from build123d import *

# Parameters (mm, degrees)
SKETCH1_R           = 3.175
BOSS_EXTRUDE1_DEPTH = 3.175
SKETCH2_R           = 14.2875
CUT_EXTRUDE1_DEPTH  = 4.175
SKETCH4_R           = 6.35
SKETCH4_R_2         = 3.175
CUT_EXTRUDE2_DEPTH  = 4.175
SKETCH8_W           = 38.1
SKETCH8_H           = 100.0125
CUT_EXTRUDE3_DEPTH  = 4.175
SKETCH10_W          = 60.325
SKETCH10_H          = 48.559243464
CUT_EXTRUDE5_DEPTH  = 4.175
FILLET2_R           = 9.525


with BuildPart() as part:
    # Sketch1 → Boss-Extrude1 (new body)
    with BuildSketch(Plane.XY):
        with BuildLine():
            Line((-35.603982701, 119.957272705), (-127, -119.957272705))
            Line((-127, -119.957272705), (127, -119.957272705))
            Line((127, -119.957272705), (35.603982701, 119.957272705))
            ThreePointArc((35.603982701, 119.957272705), (0, 144.493850724), (-35.603982701, 119.957272705))
        make_face()
        with Locations((-25.4, 106.393850724)):
            Circle(SKETCH1_R, mode=Mode.SUBTRACT)
        with Locations((25.4, 106.393850724)):
            Circle(SKETCH1_R, mode=Mode.SUBTRACT)
    extrude(amount=BOSS_EXTRUDE1_DEPTH)

    # Sketch2 → Cut-Extrude1 (cut, through all)
    with BuildSketch(Plane.XY.offset(3.175)):
        with Locations((0, 106.393850724)):
            Circle(SKETCH2_R)
    extrude(amount=-CUT_EXTRUDE1_DEPTH, mode=Mode.SUBTRACT)

    # Sketch4 → Cut-Extrude2 (cut, through all)
    with BuildSketch(Plane.XY.offset(3.175)):
        with Locations((108.571571229, -107.257272705)):
            Circle(SKETCH4_R)
        with Locations((-76.2, -107.257272705)):
            Circle(SKETCH4_R_2)
        with Locations((19.05, -107.257272705)):
            Circle(SKETCH4_R_2)
    extrude(amount=-CUT_EXTRUDE2_DEPTH, mode=Mode.SUBTRACT)

    # Sketch8 → Cut-Extrude3 (cut, through all)
    with BuildSketch(Plane(origin=(0, 0, 0), x_dir=(-1, 0, 0), z_dir=(0, 0, -1))):
        with Locations((107.95, -69.951022705)):
            Rectangle(SKETCH8_W, SKETCH8_H)
    extrude(amount=-CUT_EXTRUDE3_DEPTH, mode=Mode.SUBTRACT)

    # Sketch10 → Cut-Extrude5 (cut, through all)
    with BuildSketch(Plane.XY.offset(3.175)):
        with BuildLine():
            Line((-9.525, 69.503684351), (-9.525, -14.248029241))
            Line((-9.525, -14.248029241), (-66.344311715, -14.248029241))
            Line((-66.344311715, -14.248029241), (-29.548259348, 82.34160822))
            ThreePointArc((-29.548259348, 82.34160822), (-20.56411854, 74.320075944), (-9.525, 69.503684351))
        make_face()
        with Locations((-39.6875, -57.577650973)):
            Rectangle(SKETCH10_W, SKETCH10_H)
        Polygon((9.525, -33.298029241), (9.525, -81.857272705), (92.100213987, -81.857272705), (73.601454572, -33.298029241), align=None)
        with BuildLine():
            Line((9.525, -14.248029241), (66.344311715, -14.248029241))
            Line((66.344311715, -14.248029241), (29.548259348, 82.34160822))
            ThreePointArc((29.548259348, 82.34160822), (20.56411854, 74.320075944), (9.525, 69.503684351))
            Line((9.525, 69.503684351), (9.525, -14.248029241))
        make_face()
    extrude(amount=-CUT_EXTRUDE5_DEPTH, mode=Mode.SUBTRACT)

    # Fillet2
    fillet2_edges = [part.edges().sort_by_distance(p)[0] for p in [
        (-29.548259348, 82.34160822, 1.5875),
        (-9.525, 69.503684351, 1.5875),
        (-9.525, -14.248029241, 1.5875),
        (-66.344311715, -14.248029241, 1.5875),
        (-69.85, -33.298029241, 1.5875),
        (-9.525, -33.298029241, 1.5875),
        (-9.525, -81.857272705, 1.5875),
        (-69.85, -81.857272705, 1.5875),
        (9.525, -33.298029241, 1.5875),
        (73.601454572, -33.298029241, 1.5875),
        (92.100213987, -81.857272705, 1.5875),
        (9.525, -81.857272705, 1.5875),
        (9.525, -14.248029241, 1.5875),
        (9.525, 69.503684351, 1.5875),
        (29.548259348, 82.34160822, 1.5875),
        (66.344311715, -14.248029241, 1.5875),
    ]]
    fillet(fillet2_edges, radius=FILLET2_R)


solid = part.part
Verification items for the finished model (mm, model axes). A direction names the side the tool comes from. Coordinates: 2 decimals unless noted, no trailing zeros. Loops run counter-clockwise (first coordinate to the right, second up) from the corner with the lowest first, then second, coordinate; pieces in that order, holes last. Notation, with made-up numbers: (83.25, 39) -> (102.25, 39) arc R24 cw to (102.25, 67) -> close; hole circle Ø1 at (-18.5, 31). An arc over 180 degrees is marked (long way). Answer as a JSON object with one key per item and string values. Group by question number.
Item 1: Tool access check on faces 1 (the flat face through (-6, -15, 0)), 2 (the cylindrical face through (-28.403, 75.255, 1.565)). Record the directions out of +Z, -Z, +X, -X, +Y, -Y that give a thin tool (end or side, any length) a straight path to the whole face; none if there is none.
Item 2: Sectioned sample at D-D on y = 6.5. Record the boundary of the cut face in (x, z) (3 decimals), plus the area to 3 significant figures.
Item 3: Depth check by flat-ended pin: pin 1 (1.6 mm diameter, centred on y = -56.5, z = 2, fed in from +X); pin 2 (1 mm diameter, centred on y = 43.5, z = 1.5, fed in from -X); pin 3 (1.5 mm diameter, centred on y = -19.5, z = 1, fed in from +X). Enter the tip coordinate at first touch or a pass-through.
Item 4: Sectioned sample at B-B on x = 25.5. Record the boundary of the cut face in (y, z) (3 decimals).
Item 5: Mould release check, pull along X, two halves, no side actions. Record for faces 3 (the cylindrical face through (0.64, 144.49, 1.57)), 4 (the flat face through (81.94, -1.68, 1.57)), 5 (the flat face through (48.11, 33.62, 1.61)): +X half, -X half, draft (parallel to the pull), parting line (faces both ways), or undercut.
Item 6: Scan lines: probe 1 along Y at (x, z) = (25.4, 1.3); probe 2 along X at (y, z) = (-11, 1.3); probe 3 along X at (y, z) = (-79, 0.8). Record each from-to range of solid material in increasing order.
Item 7: Sectioned sample at C-C on x = -76.2. Record the boundary of the cut face in (y, z) (3 decimals).
Item 8: Sectioned sample at A-A on y = -50. Record the boundary of the cut face in (x, z) (3 decimals).
Evaluation:
{
 "1": {"face 1": "-Z, +X, -X, +Y, -Y", "face 2": "+Z, -Z"},
 "2": {"outline": "(-78.826, 0) -> (-58.44, 0) -> (-58.44, 3.175) -> (-78.826, 3.175) -> close; (-9.525, 0) -> (9.525, 0) -> (9.525, 3.175) -> (-9.525, 3.175) -> close; (58.44, 0) -> (78.826, 0) -> (78.826, 3.175) -> (58.44, 3.175) -> close", "area": "190 mm²"},
 "3": {"pin 1": "stops at x = 103.13", "pin 2": "stops at x = -64.92", "pin 3": "stops at x = 89.02"},
 "4": {"outline": "(-119.957, 0) -> (-81.857, 0) -> (-81.857, 3.175) -> (-119.957, 3.175) -> close; (-33.298, 0) -> (-14.248, 0) -> (-14.248, 3.175) -> (-33.298, 3.175) -> close; (75.704, 0) -> (103.22, 0) -> (103.22, 3.175) -> (75.704, 3.175) -> close; (109.567, 0) -> (134.702, 0) -> (134.702, 3.175) -> (109.567, 3.175) -> close"},
 "5": {"face 3": "parting line", "face 4": "+X half", "face 5": "undercut"},
 "6": {"probe 1": "y = -119.96 to -81.86, -33.3 to -14.25, 75.7 to 103.22, 109.57 to 134.79", "probe 2": "x = -85.49 to -59.69, -11.89 to 11.89, 59.69 to 85.49", "probe 3": "x = -88.9 to -67.13, -12.25 to 12.25, 85.08 to 111.4"},
 "7": {"outline": "(-119.957, 0) -> (-110.432, 0) -> (-110.432, 3.175) -> (-119.957, 3.175) -> close; (-104.082, 0) -> (13.393, 0) -> (13.393, 3.175) -> (-104.082, 3.175) -> close"},
 "8": {"outline": "(-88.9, 0) -> (-69.85, 0) -> (-69.85, 3.175) -> (-88.9, 3.175) -> close; (-9.525, 0) -> (9.525, 0) -> (9.525, 3.175) -> (-9.525, 3.175) -> close; (79.964, 0) -> (100.35, 0) -> (100.35, 3.175) -> (79.964, 3.175) -> close"}
}
